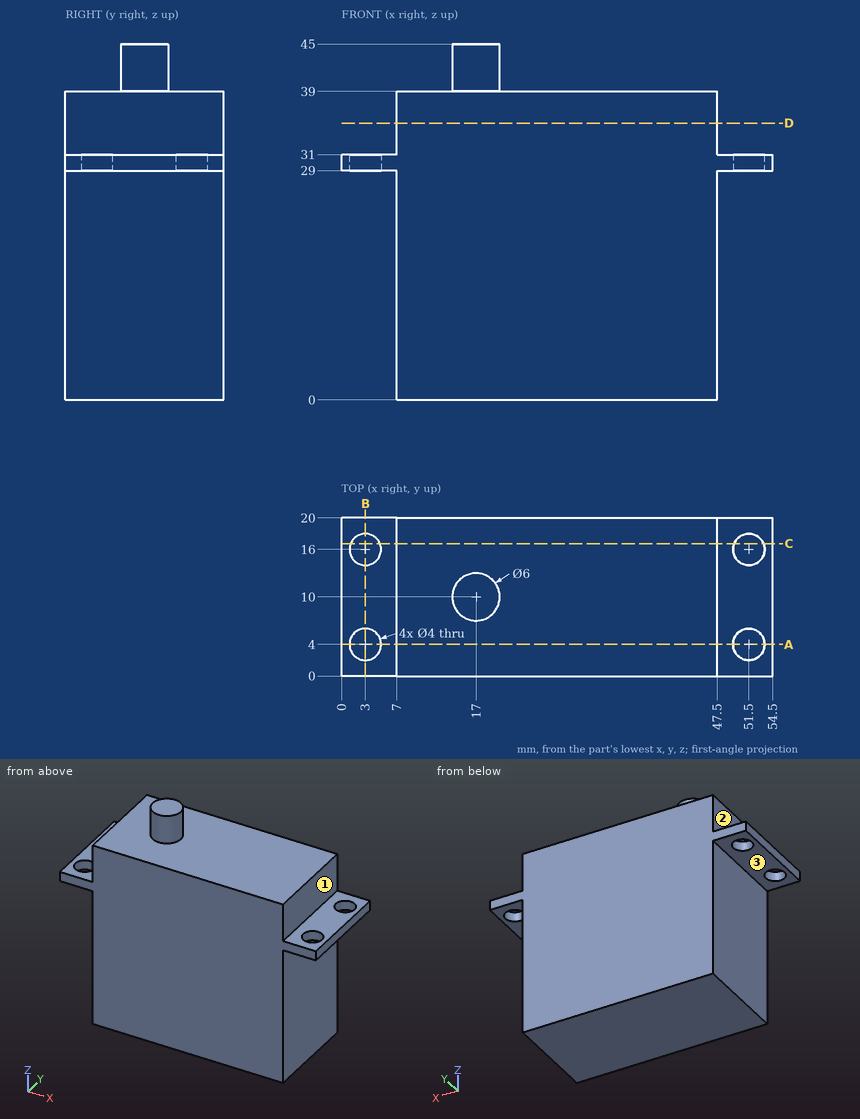
Design review of the part shown in the three views and the two pictorial views. Dimensions are in mm from the part's minimum x, y and z. A direction names the side the tool comes from. Round coordinates to 2 decimals unless told otherwise and drop trailing zeros. Write each loop counter-clockwise with the first axis right and the second up, starting at its lowest first coordinate (ties: lowest second). Pieces come first, ordered by that corner, then holes. Notation, with made-up numbers: M 86,6 L 122,6 A20 cw 122,32 Z; hole C 54,29.25 d2. An arc over 180 degrees is marked long. Use a Markdown table: item, result. Add a question column.
Q1. Insertion check: pin 1 (6.5 mm diameter, centred on x = 51.5, y = 16, fed in from +Z); pin 2 (2 mm diameter, centred on x = 4, y = 6, fed in from -Z); pin 3 (2.5 mm diameter, centred on x = 51.5, y = 4, fed in from +Z); pin 4 (5.5 mm diameter, centred on x = 49.5, y = 8, fed in from +Z). Each pin has a flat end and moves straight along its axis. Give the tip position at first contact, or say it passes through.
Q2. To check wall thickness, follow line 1 (X direction, y = 4, z = 29.55); line 2 (Y direction, x = 51.5, z = 30.4); line 3 (Y direction, x = 51, z = 30). State the ranges of each line that lie inside material, in increasing order.
Q3. We need section B-B, the plane x = 3. State the section outline as (y, z) points.
Q4. Machinability: for the marked faces 1, 2 and 3, which of the approach directions +Z, -Z, +X, -X, +Y, -Y give a long, thin tool a straight path to every point of the face, cutting with its end or side? Answer none if there is none.
Q5. We need section A-A, the plane y = 4. State the section outline as (x, z) points.
Q6. We need section D-D, the plane z = 35. State the section outline as (x, y) points.
Q7. We need section C-C, the plane y = 16.75. State the section outline as (x, z) points, plus the area to 3 significant figures.
Findings below:
| question | item | result |
|---|---|---|
| 1 | pin 1 | stops at z = 31 |
| 1 | pin 2 | stops at z = 29 |
| 1 | pin 3 | passes through |
| 1 | pin 4 | stops at z = 39 |
| 2 | line 1 | x = 0 to 1, 5 to 49.5, 53.5 to 54.5 |
| 2 | line 2 | y = 0 to 2, 6 to 14, 18 to 20 |
| 2 | line 3 | y = 0 to 2.06, 5.94 to 14.06, 17.94 to 20 |
| 3 | outline | M 0,29 L 2,29 L 2,31 L 0,31 Z; M 6,29 L 14,29 L 14,31 L 6,31 Z; M 18,29 L 20,29 L 20,31 L 18,31 Z |
| 4 | face 1 | +Z, +X, +Y, -Y |
| 4 | face 2 | +Z, -X, +Y, -Y |
| 4 | face 3 | -Z, -X, +Y, -Y |
| 5 | outline | M 0,29 L 1,29 L 1,31 L 0,31 Z; M 5,29 L 7,29 L 7,0 L 47.5,0 L 47.5,29 L 49.5,29 L 49.5,31 L 47.5,31 L 47.5,39 L 7,39 L 7,31 L 5,31 Z; M 53.5,29 L 54.5,29 L 54.5,31 L 53.5,31 Z |
| 6 | outline | M 7,0 L 47.5,0 L 47.5,20 L 7,20 Z |
| 7 | outline | M 0,29 L 1.15,29 L 1.15,31 L 0,31 Z; M 4.85,29 L 7,29 L 7,0 L 47.5,0 L 47.5,29 L 49.65,29 L 49.65,31 L 47.5,31 L 47.5,39 L 7,39 L 7,31 L 4.85,31 Z; M 53.35,29 L 54.5,29 L 54.5,31 L 53.35,31 Z |
| 7 | area | 1,590 mm² |
